Geometry check sheet. Reference: the model listing, model coordinates, mm. A direction names the side the tool comes from. Round coordinates to 2 decimals unless told otherwise and drop trailing zeros. Loops run counter-clockwise (first coordinate to the right, second up) from the corner with the lowest first, then second, coordinate; pieces in that order, holes last. Notation, with made-up numbers: M 38.5,-8.5 L 48.5,-8.5 A27 ccw 48.5,16.5 Z; hole C 19.25,72 d11. An arc over 180 degrees is marked long. Use one line per item in the form item = value. Start each with the question number.
1. Cross-section at A-A (y = -36). Record the boundary of the cut face in (x, z).
2. Cross-section at C-C (y = -5.5). Record the boundary of the cut face in (x, z), then the cut area to 3 significant figures.
3. Material ranges on line 1 (Y direction, x = -4.5, z = 1.4); line 2 (Y direction, x = 18.5, z = 5.2); line 3 (X direction, y = -16, z = 3.4), recorded low to high.
4. Cross-section at D-D (x = 6.5). Record the boundary of the cut face in (y, z).
5. Draft check along Y on faces 1 (the flat face through (6.98, -9.3, 2.96)), 2 (the flat face through (-12.694, -10, 3)), 3 (the cylindrical face through (21.65, -33.89, 2.96)). Enter one of: pulls with the +Y half, pulls with the -Y half, needs draft (parallel to the pull), parting line crosses it, or undercut.
6. Go/stop test with flat-tipped pins: pin 1 (3 mm diameter, centred on x = 5.5, z = 2, fed in from +Y); pin 2 (1.8 mm diameter, centred on y = -38.5, z = 2, fed in from -X); pin 3 (2 mm diameter, centred on x = 10, z = 3, fed in from +Y); pin 4 (1.5 mm diameter, centred on x = -4.69, y = -4.88, fed in from +Z). Record where each tip stops, or that it passes through.
7. Cross-section at B-B (z = 0.6). State how many separate pieces and enclosed holes the cut face has, then the cut area to 3 significant figures.
8. Set-up check for faces 4 (the flat face through (30.306, -30, 3)), 5 (the flat face through (-5, -19.75, 3)), 6 (the flat face through (23, -18, 3)): record each of +Z, -Z, +X, -X, +Y, -Y from which the full face is reachable in a straight line by a thin tool's end or side.
```python
from build123d import *

# Parameters (mm, degrees)
SKETCH_1_R      = 2.5
SKETCH_1_R_2    = 1.25
EXTRUDE_1_DEPTH = 6


with BuildPart() as part:
    # 草图1 → 凸台-拉伸1 (new body)
    with BuildSketch(Plane.XY):
        with BuildLine():
            Line((1.500025947, -1.999165895), (12.605850611, -16.800500463))
            ThreePointArc((12.605850611, -16.800500463), (13.664114192, -17.683421453), (15.005475182, -18))
            Line((15.005475182, -18), (30.306366751, -18))
            Line((30.306366751, -18), (30.306366751, -32.6148543))
            Line((30.306366751, -32.6148543), (30.306366751, -42))
            Line((30.306366751, -42), (10.306366751, -42))
            Line((10.306366751, -42), (10.306366751, -35.397540485))
            ThreePointArc((10.306366751, -35.397540485), (10.049618348, -33.815907061), (9.305741036, -32.39670638))
            Line((9.305741036, -32.39670638), (1.316615651, -21.749165895))
            ThreePointArc((1.316615651, -21.749165895), (-0.447156984, -20.277630912), (-2.682758634, -19.75))
            Line((-2.682758634, -19.75), (-7.693633249, -19.75))
            ThreePointArc((-7.693633249, -19.75), (-11.229167155, -18.285533906), (-12.693633249, -14.75))
            Line((-12.693633249, -14.75), (-12.693633249, -5))
            ThreePointArc((-12.693633249, -5), (-11.229167155, -1.464466094), (-7.693633249, 0))
            Line((-7.693633249, 0), (-2.499348338, 0))
            ThreePointArc((-2.499348338, 0), (-0.263746688, -0.527630912), (1.500025947, -1.999165895))
        make_face()
        with Locations((20.306366751, -36)):
            Circle(SKETCH_1_R, mode=Mode.SUBTRACT)
        with Locations((20.306366751, -24)):
            Circle(SKETCH_1_R, mode=Mode.SUBTRACT)
        with Locations((-4.693633249, -4.875)):
            Circle(SKETCH_1_R_2, mode=Mode.SUBTRACT)
        with Locations((-4.693633249, -14.875)):
            Circle(SKETCH_1_R_2, mode=Mode.SUBTRACT)
    extrude(amount=EXTRUDE_1_DEPTH)


solid = part.part
```
Reported:
q1.outline = M 10.31,0 L 17.81,0 L 17.81,6 L 10.31,6 Z; M 22.81,0 L 30.31,0 L 30.31,6 L 22.81,6 Z
q2.outline = M -12.69,0 L -5.78,0 L -5.78,6 L -12.69,6 Z; M -3.61,0 L 4.13,0 L 4.13,6 L -3.61,6 Z
q2.area = 87.9 mm²
q3.line_1 = -19.75 to -16.11, -13.64 to -6.11, -3.64 to 0
q3.line_2 = -42 to -37.73, -34.27 to -25.73, -22.27 to -18
q3.line_3 = -12.53 to -5.24, -4.15 to 12.01
q4.outline = M -28.66,0 L -8.66,0 L -8.66,6 L -28.66,6 Z
q5.face_1 = pulls with the +Y half
q5.face_2 = needs draft
q5.face_3 = undercut
q6.pin_1 = -5.33
q6.pin_2 = 10.31
q6.pin_3 = -11.99
q6.pin_4 = through
q7.separate_pieces = 1
q7.enclosed_holes = 4
q7.area = 884 mm²
q8.face_4 = +Z, -Z, +X, +Y, -Y
q8.face_5 = +Z, -Z, -X, -Y
q8.face_6 = +Z, -Z, +X, +Y
